Verification items for the finished model (mm, model axes). A direction names the side the tool comes from. Coordinates: 2 decimals unless noted, no trailing zeros. Order: outer loops, then holes, each group sorted by start corner. A loop starts at its lowest first (then second) coordinate and runs counter-clockwise, first axis right, second up. Notation, with made-up numbers: M 67,78 L 100,78 A29 ccw 100,101 Z; hole C 25,32.5 d7. An arc over 180 degrees is marked long. Return JSON: item names as keys, results as strings. Group by question number.
Q1. Mould release check, pull along Z, two halves, no side actions. Record for faces 3 (the face through (2, -5, -1)), 4 (the face through (2, -5, 1)), 5 (the face through (0, 0, 2.5)), 6 (the face through (4.72, -1.49, -17.29)): pulls with the +Z half, pulls with the -Z half, needs draft (parallel to the pull), parting line crosses it, or undercut.
Q2. Thickness scan on probe 1 along Z at (x, y) = (4.5, 3.75); probe 2 along Y at (x, z) = (5.75, 1.5); probe 3 along X at (y, z) = (-1.75, -24). Record the ranges inside material, lowest first.
Q3. Go/stop test with flat-tipped pins: pin 1 Ø1 at (x, z) = (1, -9.5) entering from +Y; pin 2 Ø4 at (x, z) = (4, -13.5) entering from -Y; pin 3 Ø4 at (x, z) = (-4.5, -26.5) entering from +Y. Record where each tip stops, or that it passes through.
Q4. Section check B-B, the plane x = 0. Enter the section's corners in (y, z), then the cut area to 3 significant figures.
Q5. Section check D-D, the plane z = -22. Enter the section's corners in (x, y).
Q6. Access from +Z, -Z, +X, -X, +Y, -Y to the whole of each face (thin tool, end or side, straight path). Record for faces 1 (the face through (0, 0, -32.5)), 2 (the face through (2, -5, -2.5)).
Q7. Section check A-A, the plane y = -6. Enter the section's corners in (x, z).
from build123d import *

# Parameters (mm, degrees)
F0_R          = 7.5
F1_DEPTH      = 2.5
F1_DEPTH_BACK = 2.5
F2_R          = 4.95
F3_DEPTH      = 30
F4_R          = 7.55
F4_R_2        = 5
F5_DEPTH      = 1
F5_DEPTH_BACK = 1


with BuildPart() as f1:
    # F0 (on Top) → F1 (new body, two sides)
    with BuildSketch(Plane.XY) as f1_sk:
        Circle(F0_R)
    extrude(amount=-F1_DEPTH)
    extrude(f1_sk.sketch, amount=F1_DEPTH_BACK)

    # F2 (on face) → F3 (join)
    with BuildSketch(Plane(origin=(0, 0, -2.5), x_dir=(1, 0, 0), z_dir=(0, 0, -1))):
        Circle(F2_R)
    extrude(amount=F3_DEPTH)

    # F4 (on Top) → F5 (cut, two sides)
    with BuildSketch(Plane.XY) as f5_sk:
        Circle(F4_R)
        Circle(F4_R_2, mode=Mode.SUBTRACT)
    extrude(amount=-F5_DEPTH, mode=Mode.SUBTRACT)
    extrude(f5_sk.sketch, amount=F5_DEPTH_BACK, mode=Mode.SUBTRACT)


solid = f1.part
Numbers:
{
 "1": {"face 3": "undercut", "face 4": "undercut", "face 5": "pulls with the +Z half", "face 6": "needs draft"},
 "2": {"probe 1": "z = -2.5 to -1, 1 to 2.5", "probe 2": "y = -4.82 to 4.82", "probe 3": "x = -4.63 to 4.63"},
 "3": {"pin 1": "stops at y = 4.92", "pin 2": "stops at y = -4.53", "pin 3": "stops at y = 4.27"},
 "4": {"outline": "M -7.5,-2.5 L -4.95,-2.5 L -4.95,-32.5 L 4.95,-32.5 L 4.95,-2.5 L 7.5,-2.5 L 7.5,-1 L 5,-1 L 5,1 L 7.5,1 L 7.5,2.5 L -7.5,2.5 L -7.5,1 L -5,1 L -5,-1 L -7.5,-1 Z", "area": "362 mm2"},
 "5": {"outline": "C 0,0 d9.9"},
 "6": {"face 1": "-Z, +X, -X, +Y, -Y", "face 2": "-Z"},
 "7": {"outline": "M -4.5,-2.5 L 4.5,-2.5 L 4.5,-1 L -4.5,-1 Z; M -4.5,1 L 4.5,1 L 4.5,2.5 L -4.5,2.5 Z"}
}
